```python
from build123d import *

# Parameters (mm, degrees)
SKETCH1_W           = 180
SKETCH1_H           = 230
BOSS_EXTRUDE1_DEPTH = 3
FILLET1_R           = 10
SKETCH2_R           = 1.7
CUT_EXTRUDE1_DEPTH  = 3
SKETCH3_R           = 1.7
CUT_EXTRUDE2_DEPTH  = 3
SKETCH7_W           = 30
SKETCH7_H           = 80
CUT_EXTRUDE7_DEPTH  = 167.460205455
CUT_EXTRUDE8_DEPTH  = 167.460205455


with BuildPart() as part:
    # Sketch1 → Boss-Extrude1 (new body)
    with BuildSketch(Plane(origin=(0, 0, 0), x_dir=(1, 0, 0), z_dir=(0, 1, 0))):
        with Locations((0, 25)):
            Rectangle(SKETCH1_W, SKETCH1_H)
    extrude(amount=BOSS_EXTRUDE1_DEPTH)

    # Fillet1
    fillet1_edges = [part.edges().sort_by_distance(p)[0] for p in [
        (90, 1.5, 90),
        (-90, 1.5, 90),
        (-90, 1.5, -140),
        (90, 1.5, -140),
    ]]
    fillet(fillet1_edges, radius=FILLET1_R)

    # Sketch2 → Cut-Extrude1 (cut)
    with BuildSketch(Plane(origin=(0, 3, 0), x_dir=(1, 0, 0), z_dir=(0, 1, 0))):
        with Locations(Location((-82, 120, 0), (0, 0, 270))):
            Circle(SKETCH2_R)
        with Locations(Location((-68, 120, 0), (0, 0, 270))):
            Circle(SKETCH2_R)
        with Locations(Location((68, 120, 0), (0, 0, 270))):
            Circle(SKETCH2_R)
        with Locations(Location((82, 120, 0), (0, 0, 270))):
            Circle(SKETCH2_R)
        with Locations(Location((-82, -75, 0), (0, 0, 270))):
            Circle(SKETCH2_R)
        with Locations(Location((-68, -75, 0), (0, 0, 270))):
            Circle(SKETCH2_R)
        with Locations(Location((68, -75, 0), (0, 0, 270))):
            Circle(SKETCH2_R)
        with Locations(Location((82, -75, 0), (0, 0, 270))):
            Circle(SKETCH2_R)
        with Locations(Location((-67, -30, 0), (0, 0, 270))):
            Circle(SKETCH2_R)
        with Locations(Location((-67, -46, 0), (0, 0, 270))):
            Circle(SKETCH2_R)
        with Locations(Location((-53, -30, 0), (0, 0, 270))):
            Circle(SKETCH2_R)
        with Locations(Location((-53, -46, 0), (0, 0, 270))):
            Circle(SKETCH2_R)
        with Locations(Location((53, -30, 0), (0, 0, 270))):
            Circle(SKETCH2_R)
        with Locations(Location((53, -46, 0), (0, 0, 270))):
            Circle(SKETCH2_R)
        with Locations(Location((67, -30, 0), (0, 0, 270))):
            Circle(SKETCH2_R)
        with Locations(Location((67, -46, 0), (0, 0, 270))):
            Circle(SKETCH2_R)
        with Locations(Location((-54, -75, 0), (0, 0, 270))):
            Circle(SKETCH2_R)
        with Locations(Location((54, -75, 0), (0, 0, 270))):
            Circle(SKETCH2_R)
        with Locations(Location((-40, -75, 0), (0, 0, 270))):
            Circle(SKETCH2_R)
        with Locations(Location((40, -75, 0), (0, 0, 270))):
            Circle(SKETCH2_R)
    extrude(amount=-CUT_EXTRUDE1_DEPTH, mode=Mode.SUBTRACT)

    # Sketch3 → Cut-Extrude2 (cut)
    with BuildSketch(Plane(origin=(0, 3, 0), x_dir=(1, 0, 0), z_dir=(0, 1, 0))):
        with Locations(Location((10, 75, 0), (0, 0, 270))):
            Circle(SKETCH3_R)
        with Locations(Location((-10, 75, 0), (0, 0, 270))):
            Circle(SKETCH3_R)
        with Locations(Location((-10, 115, 0), (0, 0, 270))):
            Circle(SKETCH3_R)
        with Locations(Location((10, 115, 0), (0, 0, 270))):
            Circle(SKETCH3_R)
    extrude(amount=-CUT_EXTRUDE2_DEPTH, mode=Mode.SUBTRACT)

    # Sketch7 → Cut-Extrude7 (cut, through all)
    with BuildSketch(Plane(origin=(0, 3, 0), x_dir=(1, 0, 0), z_dir=(0, 1, 0))):
        with Locations((-90, -38)):
            Rectangle(SKETCH7_W, SKETCH7_H)
        with Locations((90, -38.099840659)):
            Rectangle(SKETCH7_W, SKETCH7_H)
    extrude(amount=-CUT_EXTRUDE7_DEPTH, mode=Mode.SUBTRACT)

    # Sketch8 → Cut-Extrude8 (cut, through all)
    with BuildSketch(Plane(origin=(0, 3, 0), x_dir=(1, 0, 0), z_dir=(0, 1, 0))):
        with BuildLine():
            Line((-35, 47.5), (35, 47.5))
            ThreePointArc((35, 47.5), (42.5, 40), (35, 32.5))
            Line((35, 32.5), (-35, 32.5))
            ThreePointArc((-35, 32.5), (-42.5, 40), (-35, 47.5))
        make_face()
        with BuildLine():
            Line((-35, 7.5), (35, 7.5))
            ThreePointArc((35, 7.5), (42.5, 0), (35, -7.5))
            Line((35, -7.5), (-35, -7.5))
            ThreePointArc((-35, -7.5), (-42.5, 0), (-35, 7.5))
        make_face()
        with BuildLine():
            Line((-57.5, 97.5), (-57.5, 52.5))
            ThreePointArc((-57.5, 52.5), (-62.5, 47.5), (-67.5, 52.5))
            Line((-67.5, 52.5), (-67.5, 97.5))
            ThreePointArc((-67.5, 97.5), (-62.5, 102.5), (-57.5, 97.5))
        make_face()
        with BuildLine():
            Line((67.5, 97.5), (67.5, 52.5))
            ThreePointArc((67.5, 52.5), (62.5, 47.5), (57.5, 52.5))
            Line((57.5, 52.5), (57.5, 97.5))
            ThreePointArc((57.5, 97.5), (62.5, 102.5), (67.5, 97.5))
        make_face()
    extrude(amount=-CUT_EXTRUDE8_DEPTH, mode=Mode.SUBTRACT)


solid = part.part
```
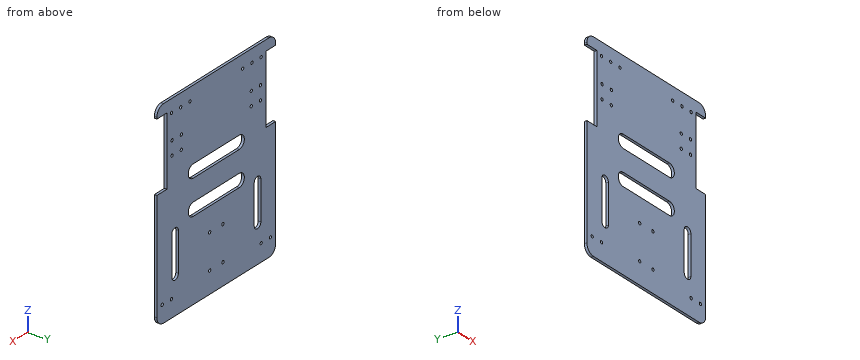
CAD build for the part. Positions are in the model's coordinates, mm. Round coordinates to 2 decimals unless told otherwise and drop trailing zeros. Write each loop counter-clockwise with the first axis right and the second up, starting at its lowest first coordinate (ties: lowest second). Pieces come first, ordered by that corner, then holes. Notation, with made-up numbers: (15, -19.5) - (40, -19.5) arc R16 ccw to (40, -15.5) - close; hole circle Ø5 at (80.5, -3). An arc over 180 degrees is marked (long way). Return JSON: item names as keys, results as strings. Group by question number.
Item 1: Probe probe 1 along Z at (x, y) = (18, 2.6); probe 2 along X at (y, z) = (1.9, 46); probe 3 along Z at (x, y) = (-76, 0.7). List the from-to ranges inside material, lowest first.
Item 2: Band-saw the part on C-C on x = 62.5. List the corners of the cut face in (y, z), plus the area to 3 significant figures.
Item 3: Band-saw the part on B-B on z = -57. List the corners of the cut face in (x, y).
Item 4: Flat gauge pins, fed straight in: pin 1 Ø3 at (x, z) = (-53, 46) entering from -Y; pin 2 Ø0.9 at (x, y) = (83, 2) entering from -Z; pin 3 Ø4 at (x, z) = (-53, 30) entering from -Y; pin 4 Ø0.9 at (x, y) = (-82, 1.5) entering from +Z. Where does each tip first touch, or does it go through?
Item 5: Band-saw the part on D-D on y = 1.25. State how many separate pieces and enclosed holes the cut face has, plus the area to 3 significant figures.
Item 6: Band-saw the part on A-A on x = 26.5. List the corners of the cut face in (y, z).
Resolved:
{
 "1": {"probe 1": "z = -140 to -47.5, -32.5 to -7.5, 7.5 to 90", "probe 2": "x = -75 to -68.7, -65.3 to -54.7, -51.3 to 51.3, 54.7 to 65.3, 68.7 to 75", "probe 3": "z = -140 to -2, 78 to 90"},
 "2": {"outline": "(0, -140) - (3, -140) - (3, -102.5) - (0, -102.5) - close; (0, -47.5) - (3, -47.5) - (3, 90) - (0, 90) - close", "area": "525 mm²"},
 "3": {"outline": "(-90, 0) - (-67.5, 0) - (-67.5, 3) - (-90, 3) - close; (-57.5, 0) - (57.5, 0) - (57.5, 3) - (-57.5, 3) - close; (67.5, 0) - (90, 0) - (90, 3) - (67.5, 3) - close"},
 "4": {"pin 1": "passes through", "pin 2": "stops at z = -139.67", "pin 3": "stops at y = 0", "pin 4": "stops at z = 89.88"},
 "5": {"separate pieces": "1", "enclosed holes": "26", "area": "35,200 mm²"},
 "6": {"outline": "(0, -140) - (3, -140) - (3, -47.5) - (0, -47.5) - close; (0, -32.5) - (3, -32.5) - (3, -7.5) - (0, -7.5) - close; (0, 7.5) - (3, 7.5) - (3, 90) - (0, 90) - close"}
}
